from build123d import *

# Parameters (mm, degrees)
F0_R     = 80
F0_R_2   = 10
F1_DEPTH = 25
F2_R     = 7.5
F3_DEPTH = 35
F4_R     = 7.5
F4_R_2   = 11.25
F5_DEPTH = 17.5


with BuildPart() as f1:
    # F0 (on Top) → F1 (new body)
    with BuildSketch(Plane.XY):
        Circle(F0_R)
        Circle(F0_R_2, mode=Mode.SUBTRACT)
    extrude(amount=F1_DEPTH)

    # F2 (on face) → F3 (join)
    with BuildSketch(Plane.XY.offset(25)):
        with Locations((0, 60)):
            Circle(F2_R)
    extrude(amount=F3_DEPTH)

    # F4 (on face) → F5 (join)
    with BuildSketch(Plane.XY.offset(25)):
        with Locations((0, 60)):
            Circle(F4_R)
        with Locations((0, 60)):
            Circle(F4_R_2)
        with Locations((0, 60)):
            Circle(F4_R, mode=Mode.SUBTRACT)
    extrude(amount=F5_DEPTH)


solid = f1.part
Design review of the part built by this model. Coordinates are the model's own, in mm. A direction names the side the tool comes from. Coordinates: 2 decimals unless noted, no trailing zeros. Loops run counter-clockwise (first coordinate to the right, second up) from the corner with the lowest first, then second, coordinate; pieces in that order, holes last. Notation, with made-up numbers: (47.25, 36) - (101.25, 36) arc R11 cw to (101.25, 41) - close; hole circle Ø2 at (51, 32.25). An arc over 180 degrees is marked (long way). Use CSV: the item, a comma, the result in double quotes. Start each with the question number.
1. To check wall thickness, follow probe 1 along Y at (x, z) = (0, 11); probe 2 along Z at (x, y) = (31.5, 8.5); probe 3 along Y at (x, z) = (33, 15). State the ranges of each line that lie inside material, in increasing order.
2. Add section C-C on z = 16. Give the boundary of the cut face in (x, y), plus the area to 3 significant figures.
3. Add section D-D on y = 56.5. Give the boundary of the cut face in (x, z), plus the area to 3 significant figures.
4. For faces 4 (the flat face through (7.3, 57.7, 42.5)), 5 (the flat face through (0, 60, 60)), list the 3-axis set-ups (+Z, -Z, +X, -X, +Y, -Y) from which the entire face can be reached by the end or side of a thin tool; tool diameter is ignored.
5. Clearance check with flat-ended pins moving along their axes: pin 1 (1.5 mm diameter, centred on x = -46.5, y = -13.5, fed in from +Z); pin 2 (4 mm diameter, centred on y = 60, z = 21.5, fed in from +X); pin 3 (10 mm diameter, centred on y = 26, z = 25, fed in from -X). State where each tip first meets the part, or that it passes through.
6. Add section A-A on y = 0. Give the boundary of the cut face in (x, z), plus the area to 3 significant figures.
7. Add section B-B on x = -5.5. Give the boundary of the cut face in (y, z).
8. Mouldability with a two-part tool opening along Y and no side actions: class faces 1 (the cylindrical face through (-2.17, -9.76, 12.32)), 2 (the flat face through (17, 1, 0)), 3 (the cylindrical face through (-1.465, 71.154, 33.628)) as released by +Y, released by -Y, zero draft, split by the parting line, or undercut.
Resolved:
1,probe 1,"-80 to -10, 10 to 80"
1,probe 2,"0 to 25"
1,probe 3,"-72.88 to 72.88"
2,outline,"circle Ø160 at (0, 0); hole circle Ø20 at (0, 0)"
2,area,"19,800 mm2"
3,outline,"(-56.64, 0) - (56.64, 0) - (56.64, 25) - (10.69, 25) - (10.69, 42.5) - (6.63, 42.5) - (6.63, 60) - (-6.63, 60) - (-6.63, 42.5) - (-10.69, 42.5) - (-10.69, 25) - (-56.64, 25) - close"
3,area,"3,440 mm2"
4,face 4,"+Z"
4,face 5,"+Z, +X, -X, +Y, -Y"
5,pin 1,"z = 25"
5,pin 2,"x = 55.1"
5,pin 3,"x = -77.19"
6,outline,"(-80, 0) - (-10, 0) - (-10, 25) - (-80, 25) - close; (10, 0) - (80, 0) - (80, 25) - (10, 25) - close"
6,area,"3,500 mm2"
7,outline,"(-79.81, 0) - (-8.35, 0) - (-8.35, 25) - (-79.81, 25) - close; (8.35, 0) - (79.81, 0) - (79.81, 25) - (69.81, 25) - (69.81, 42.5) - (65.1, 42.5) - (65.1, 60) - (54.9, 60) - (54.9, 42.5) - (50.19, 42.5) - (50.19, 25) - (8.35, 25) - close"
8,face 1,"undercut"
8,face 2,"zero draft"
8,face 3,"split by the parting line"
